```python
from build123d import *

# Parameters (mm, degrees)
SKETCH008_R        = 5.130378
PAD006_DEPTH       = 1.2
PAD004_DEPTH       = 2
PAD005_DEPTH       = 3.5
POCKET_DEPTH       = 2.25
SKETCH009_R        = 3.757957
POCKET003002_DEPTH = 5


with BuildPart() as servo_support_cylinder001:
    # Sketch008 → Pad006 (new body)
    with BuildSketch(Plane.XY.offset(26.7)):
        Circle(SKETCH008_R)
    extrude(amount=PAD006_DEPTH)


with BuildPart() as servo_leg:
    # Sketch005 → Pad004 (new body, symmetric)
    with BuildSketch(Plane.XZ):
        with BuildLine():
            Line((-5.48246, 27.836502), (19.959321, 27.836502))
            ThreePointArc((27.493431, 21.408161), (24.91125, 26.011021), (19.959321, 27.836502))
            Line((27.493431, 21.408161), (30.905711, 0))
            Line((33.905711, 0), (30.905711, 0))
            Line((31.140427, 21.501308), (33.905711, 0))
            ThreePointArc((31.140427, 21.501308), (27.404927, 28.527815), (19.959321, 31.336502))
            Line((-5.48246, 31.336502), (19.959321, 31.336502))
            Line((-5.48246, 27.836502), (-5.48246, 31.336502))
        make_face()
    extrude(amount=PAD004_DEPTH, both=True)

    # Sketch006 → Pad005 (new body)
    with BuildSketch(Plane(origin=(0, 0, 31.336502), x_dir=(-1, 0, 0), z_dir=(0, 0, 1))):
        with BuildLine():
            Line((-19.908253, 1.9951), (0, 6.517084))
            ThreePointArc((6.517084, 0), (4.608274, 4.608274), (0, 6.517084))
            Line((6.517084, 0), (0, 0))
            Line((-19.908253, 0), (0, 0))
            Line((-19.908253, 1.9951), (-19.908253, 0))
        make_face()
    pad005 = extrude(amount=-PAD005_DEPTH)

    # Mirrored: Pad005 across Sketch006 H_Axis
    add(pad005.mirror(Plane(origin=(0, 0, 31.336502), x_dir=(0, 0, 1), z_dir=(0, -1, 0))))

    # Sketch007 → Pocket (cut)
    with BuildSketch(Plane(origin=(0, 0, 31.336502), x_dir=(-1, 0, 0), z_dir=(0, 0, 1))):
        with BuildLine():
            Line((-18.037807, 1.500282), (0, 4.25))
            ThreePointArc((2e-06, -4.25), (4.25, 1e-06), (0, 4.25))
            Line((-18.038573, -1.499718), (2e-06, -4.25))
            ThreePointArc((-18.037807, 1.500282), (-18.79662, 0.000476), (-18.038573, -1.499718))
        make_face()
    extrude(amount=-POCKET_DEPTH, mode=Mode.SUBTRACT)

    # Fusion007002: union servo_support_cylinder001
    add(servo_support_cylinder001.part)

    # Sketch009 → Pocket003002 (cut)
    with BuildSketch(Plane(origin=(0, 0, 26.7), x_dir=(1, 0, 0), z_dir=(0, 0, -1))):
        Circle(SKETCH009_R)
    extrude(amount=-POCKET003002_DEPTH, mode=Mode.SUBTRACT)


solid = servo_leg.part
```
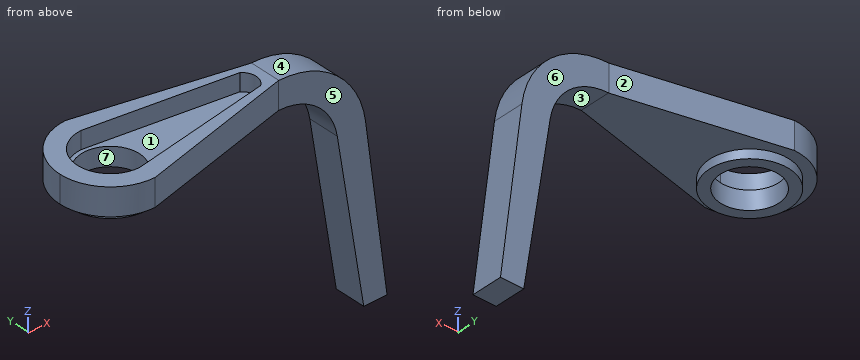
Verification items for the finished model (mm, model axes). Face numbers are marked on the shaded views. A direction names the side the tool comes from. Coordinates: 2 decimals unless noted, no trailing zeros. Loops run counter-clockwise (first coordinate to the right, second up) from the corner with the lowest first, then second, coordinate; pieces in that order, holes last. Notation, with made-up numbers: (-4.5, 15.25) -> (50.5, 15.25) arc R24 ccw to (50.5, 44.25) -> close; hole circle Ø8 at (-26, -24.75). An arc over 180 degrees is marked (long way). Answer in a Markdown table with one row per item.
1) Access from +Z, -Z, +X, -X, +Y, -Y to the whole of each face (thin tool, end or side, straight path). Record for the marked faces 1, 2 and 3.
The answers:
| item | result |
|---|---|
| face 1 | +Z |
| face 2 | +Z, -Z, +X, +Y |
| face 3 | -Z, +Y, -Y |
2) Depth check by flat-ended pin: P1, Ø15.5, axis at x = 29.5, z = 17, coming from the +Y side; P2, Ø6.5, axis at x = 6.5, y = -3, coming from the -Z side; P3, Ø5, axis at x = 11, y = 0, coming from the +Z side. Enter the tip coordinate at first touch or a pass-through.
The answers:
| item | result |
|---|---|
| P1 | stops at y = 2 |
| P2 | stops at z = 26.7 |
| P3 | stops at z = 29.09 |
3) Draft check along Y on the marked faces 4, 5, 6 and 7. Enter one of: released by +Y, released by -Y, zero draft, split by the parting line, or undercut.
The answers:
| item | result |
|---|---|
| face 4 | zero draft |
| face 5 | released by -Y |
| face 6 | released by +Y |
| face 7 | undercut |
4) Scan lines: line 1 along Y through (x, z) = (0, 28.6); line 2 along X through (y, z) = (0, 27.2); line 3 along Y through (x, z) = (0, 27.35). Record each from-to range of solid material in increasing order. Write a range as from..to.
The answers:
| item | result |
|---|---|
| line 1 | y = -6.52..-3.76, 3.76..6.52 |
| line 2 | x = -5.13..-3.76, 3.76..5.13, 23.01..28.69 |
| line 3 | y = -5.13..-3.76, 3.76..5.13 |
5) Section check C-C (x = 28.5). Record the cut outline in (y, z), and give its area (3 significant figures).
The answers:
| item | result |
|---|---|
| outline | (-2, 15.09) -> (2, 15.09) -> (2, 27.42) -> (-2, 27.42) -> close |
| area | 49.3 mm2 |
6) Section check B-B (z = 23). Record the cut outline in (x, y), and give its area (3 significant figures).
The answers:
| item | result |
|---|---|
| outline | (27.06, -2) -> (30.84, -2) -> (30.84, 2) -> (27.06, 2) -> close |
| area | 15.1 mm2 |
7) Section check A-A (x = 13.5). Record the cut outline in (y, z).
The answers:
| item | result |
|---|---|
| outline | (-3.45, 27.84) -> (3.45, 27.84) -> (3.45, 31.34) -> (2.19, 31.34) -> (2.19, 29.09) -> (-2.19, 29.09) -> (-2.19, 31.34) -> (-3.45, 31.34) -> close |
